For this review, take the finished solid that the model builds, in its own axes (mm). A direction names the side the tool comes from. Coordinates: 2 decimals unless noted, no trailing zeros. Loops run counter-clockwise (first coordinate to the right, second up) from the corner with the lowest first, then second, coordinate; pieces in that order, holes last. Notation, with made-up numbers: M -25,31 L -14,31 A7 ccw -14,39 Z; hole C 7,-34.5 d10. An arc over 180 degrees is marked long. Write each question's results on one line, items separated by ' | '. Start each with the question number.
```python
from build123d import *

# Parameters (mm, degrees)
SKETCH1_R           = 6.5
BOSS_EXTRUDE1_DEPTH = 5
SKETCH2_R           = 1.6
BOSS_EXTRUDE2_DEPTH = 3


with BuildPart() as part:
    # Sketch1 → Boss-Extrude1 (new body)
    with BuildSketch(Plane.XY):
        with BuildLine():
            Line((-9.5, 0), (-9.5, 9.5))
            Line((-9.5, 9.5), (9.5, 9.5))
            Line((9.5, 9.5), (9.5, 0))
            ThreePointArc((9.5, 0), (0, -9.5), (-9.5, 0))
        make_face()
        Circle(SKETCH1_R, mode=Mode.SUBTRACT)
    extrude(amount=BOSS_EXTRUDE1_DEPTH)

    # Sketch2 → Boss-Extrude2 (add)
    with BuildSketch(Plane(origin=(0, 9.5, 0), x_dir=(1, 0, 0), z_dir=(0, 1, 0))):
        with BuildLine():
            Line((13.1, 1.1), (-13.1, 1.1))
            ThreePointArc((-13.1, 1.1), (-16.7, -2.5), (-13.1, -6.1))
            Line((-13.1, -6.1), (13.1, -6.1))
            ThreePointArc((13.1, -6.1), (16.7, -2.5), (13.1, 1.1))
        make_face()
        with Locations((-13.1, -2.5)):
            Circle(SKETCH2_R, mode=Mode.SUBTRACT)
        with Locations((13.1, -2.5)):
            Circle(SKETCH2_R, mode=Mode.SUBTRACT)
    extrude(amount=BOSS_EXTRUDE2_DEPTH)


solid = part.part
```
Q1. The part is to be moulded in two halves that separate along Y. For faces 1 (the face through (-2, 6.5, 5)), 2 (the face through (-5.158, -3.955, 2.465)), 3 (the face through (0.209, -9.498, 2.465)), say which applies: pulls with the +Y half, pulls with the -Y half, needs draft (parallel to the pull), parting line crosses it, or undercut.
Q2. To check wall thickness, follow line 1 along X through (y, z) = (10.9, 2.5); line 2 along Z through (x, y) = (13.1, 10.8); line 3 along Y through (x, z) = (0, 2.2). State the ranges of each line that lie inside material, in increasing order.
Q3. Insertion check: P1, Ø9.5, axis at x = 1.5, y = 2.5, coming from the +Z side; P2, Ø1, axis at y = 2, z = 2.5, coming from the +X side; P3, Ø4, axis at x = -5, y = 8.5, coming from the +Z side; P4, Ø4, axis at x = 13.1, z = 2.5, coming from the -Y side. Each pin has a flat end and moves straight along its axis. Give the tip position at first contact, or say it passes through.
Q4. Take a section at D-D, the plane y = -5.75. Give the boundary of the cut face in (x, z).
Q5. For faces 4 (the face through (-2, 6.5, 0)), 5 (the face through (9.5, 5, 2)), 6 (the face through (-9.5, 5, 2)), list the 3-axis set-ups (+Z, -Z, +X, -X, +Y, -Y) from which the entire face can be reached by the end or side of a thin tool; tool diameter is ignored.
Q6. Take a section at A-A, the plane z = 2.5. Give the boundary of the cut face in (x, y).
Q7. Take a section at C-C, the plane y = 6. Give the boundary of the cut face in (x, z).
Q8. Take a section at B-B, the plane x = 0. Give the boundary of the cut face in (y, z), then the cut area to 3 significant figures.
Results:
1) face 1: needs draft | face 2: undercut | face 3: pulls with the -Y half
2) line 1: -16.7 to -14.7, -11.5 to 11.5, 14.7 to 16.7 | line 2: -1.1 to 0.9, 4.1 to 6.1 | line 3: -9.5 to -6.5, 6.5 to 12.5
3) P1: z = 5 | P2: x = 9.5 | P3: z = 6.1 | P4: y = 9.5
4) outline: M -7.56,0 L -3.03,0 L -3.03,5 L -7.56,5 Z; M 3.03,0 L 7.56,0 L 7.56,5 L 3.03,5 Z
5) face 4: -Z, +X, -X, -Y | face 5: +Z, -Z, +X, -Y | face 6: +Z, -Z, -X, -Y
6) outline: M -16.7,9.5 L -14.7,9.5 L -14.7,12.5 L -16.7,12.5 Z; M -11.5,9.5 L -9.5,9.5 L -9.5,0 A9.5 ccw 9.5,0 L 9.5,9.5 L 11.5,9.5 L 11.5,12.5 L -11.5,12.5 Z; M 14.7,9.5 L 16.7,9.5 L 16.7,12.5 L 14.7,12.5 Z; hole C 0,0 d13
7) outline: M -9.5,0 L -2.5,0 L -2.5,5 L -9.5,5 Z; M 2.5,0 L 9.5,0 L 9.5,5 L 2.5,5 Z
8) outline: M -9.5,0 L -6.5,0 L -6.5,5 L -9.5,5 Z; M 6.5,0 L 9.5,0 L 9.5,-1.1 L 12.5,-1.1 L 12.5,6.1 L 9.5,6.1 L 9.5,5 L 6.5,5 Z | area: 51.6 mm^2
